```python
from build123d import *

# Parameters (mm, degrees)
PAD_DEPTH = 65
FILLET_R  = 4


with BuildPart() as part:
    # Sketch → Pad (new body)
    with BuildSketch(Plane.XZ):
        Polygon((-60, 103.923048), (0, 0), (-60, 0), (-60, 10), (-15.773503, 10), (-70, 103.923048), align=None)
    extrude(amount=PAD_DEPTH)

    # Fillet
    fillet_edges = [part.edges().sort_by_distance(p)[0] for p in [
        (0, -32.5, 0),
        (-60, -32.5, 0),
        (-60, -32.5, 10),
        (-70, -32.5, 103.923048),
        (-60, -32.5, 103.923048),
    ]]
    fillet(fillet_edges, radius=FILLET_R)


solid = part.part
```
Here's how the part is built. I have some questions about the finished solid (model axes, mm). A direction names the side the tool comes from. Coordinates: 2 decimals unless noted, no trailing zeros. Write each loop counter-clockwise with the first axis right and the second up, starting at its lowest first coordinate (ties: lowest second). Pieces come first, ordered by that corner, then holes. Notation, with made-up numbers: (39.25, -20.75) -> (91.25, -20.75) arc R9 cw to (91.25, -12.75) -> close; hole circle Ø7 at (53.25, 2). An arc over 180 degrees is marked (long way). Use a Markdown table: item, result. Add a question column.
(1) Please list where these lines run through material, in increasing order: line 1 (Z direction, x = -16.5, y = -17.5); line 2 (Z direction, x = -26, y = -15); line 3 (X direction, y = -20.5, z = 4).
(2) If we section it at C-C, the plane z = 16: Write out the boundary of the cut face in (x, y), and give its area (3 significant figures).
(3) We'd pull the mould along Z, two halves only. Please class faces 1 (the flat face through (-30, -65, 37)), 2 (the flat face through (-31, -32, 0)), 3 (the flat face through (-36, -32, 10)): +Z half, -Z half, draft (parallel to the pull), parting line (faces both ways), or undercut.
(4) If we section it at D-D, the plane x = -13: Write out the boundary of the cut face in (y, z).
(5) I'm going to push flat-ended pins straight in: P1, Ø2, axis at y = -37.5, z = 5, coming from the -X side; P2, Ø20, axis at x = -39.5, y = -26.5, coming from the +Z side; P3, Ø2, axis at y = -16.5, z = 41, coming from the +X side. Where does each tip first touch, or does it pass through?
(6) If we section it at B-B, the plane x = -21: Write out the boundary of the cut face in (y, z), and give its area (3 significant figures).
(7) If we section it at A-A, the plane y = -55.5: Write out the boundary of the cut face in (x, z), and give its area (3 significant figures).
(8) For faces 4 (the flat face through (-30, 0, 37)), 5 (the cylindrical face through (-58.859, -32.955, 8.797)), which set-ups out of +Z, -Z, +X, -X, +Y, -Y let a thin tool reach every point of the face, with its end or its side?
Outcome:
| question | item | result |
|---|---|---|
| 1 | line 1 | z = 0 to 10, 11.26 to 28.58 |
| 1 | line 2 | z = 0 to 10, 27.71 to 45.03 |
| 1 | line 3 | x = -60 to -2.93 |
| 2 | outline | (-19.24, -65) -> (-9.24, -65) -> (-9.24, 0) -> (-19.24, 0) -> close |
| 2 | area | 650 mm^2 |
| 3 | face 1 | draft |
| 3 | face 2 | -Z half |
| 3 | face 3 | undercut |
| 4 | outline | (-65, 0) -> (0, 0) -> (0, 22.52) -> (-65, 22.52) -> close |
| 5 | P1 | stops at x = -60 |
| 5 | P2 | stops at z = 85.74 |
| 5 | P3 | stops at x = -23.09 |
| 6 | outline | (-65, 0) -> (0, 0) -> (0, 10) -> (-65, 10) -> close; (-65, 19.05) -> (0, 19.05) -> (0, 36.37) -> (-65, 36.37) -> close |
| 6 | area | 1,780 mm^2 |
| 7 | outline | (-66.54, 97.92) -> (-15.77, 10) -> (-56, 10) arc R4 ccw to (-60, 6) -> (-60, 4) arc R4 ccw to (-56, 0) -> (-6.93, 0) arc R4 ccw to (-3.46, 6) -> (-58.85, 101.92) arc R4 ccw to (-62.31, 103.92) -> (-63.07, 103.92) arc R4 ccw to start |
| 7 | area | 1,480 mm^2 |
| 8 | face 4 | +Z, -Z, +X, -X, +Y |
| 8 | face 5 | -X, +Y, -Y |
